For this review, take the finished solid that the model builds, in its own axes (mm). Face numbers are marked on the shaded views. A direction names the side the tool comes from. Coordinates: 2 decimals unless noted, no trailing zeros. Write each loop counter-clockwise with the first axis right and the second up, starting at its lowest first coordinate (ties: lowest second). Pieces come first, ordered by that corner, then holes. Notation, with made-up numbers: M 59,8.25 L 112,8.25 A23 ccw 112,30.25 Z; hole C 69.5,78 d11. An arc over 180 degrees is marked long. One line per question, with ' | ' between items.
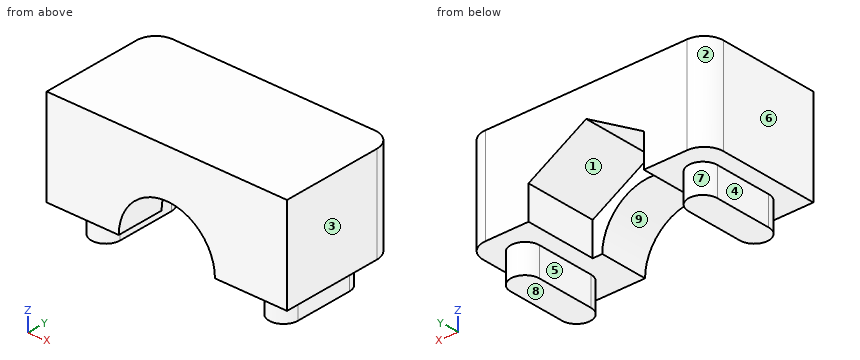
from build123d import *

# Parameters (mm, degrees)
BOSS_EXTRU_1_DEPTH      = 12.5
BOSS_EXTRU_1_DEPTH_BACK = 12.5
ESQUISSE3_W             = 25
ESQUISSE3_H             = 10
BOSS_EXTRU_2_DEPTH      = 12.5
ENL_V_MAT_EXTRU_3_DEPTH = 7.5
ESQUISSE5_R             = 5
ENL_V_MAT_EXTRU_4_DEPTH = 6
ESQUISSE6_W             = 73.841898386
ESQUISSE6_H             = 62.78176119
ENL_V_MAT_EXTRU_5_DEPTH = 26
BOSS_EXTRU_3_DEPTH      = 3
CONG_1_R                = 2


with BuildPart() as part:
    # Esquisse1 → Boss.-Extru.1 (new body, two sides)
    with BuildSketch(Plane(origin=(0, 0, 0), x_dir=(1, 0, 0), z_dir=(0, 1, 0))) as boss_extru_1_sk:
        with BuildLine():
            Line((-3, 21), (-3, -21))
            ThreePointArc((-3, -21), (-4.464466094, -24.535533906), (-8, -26))
            Line((-8, -26), (-63, -26))
            Line((-63, -26), (-63, -29))
            Line((-63, -29), (-3, -29))
            Line((-3, -29), (0, -29))
            Line((0, -29), (0, 29))
            Line((0, 29), (-3, 29))
            Line((-3, 29), (-63, 29))
            Line((-63, 29), (-63, 26))
            Line((-63, 26), (-8, 26))
            ThreePointArc((-8, 26), (-4.464466094, 24.535533906), (-3, 21))
        make_face()
    extrude(amount=BOSS_EXTRU_1_DEPTH)
    extrude(boss_extru_1_sk.sketch, amount=-BOSS_EXTRU_1_DEPTH_BACK)

    # Esquisse3 → Boss.-Extru.2 (add)
    with BuildSketch(Plane(origin=(0, 0, 0), x_dir=(1, 0, 0), z_dir=(0, 1, 0))):
        with Locations((-12.5, 34)):
            Rectangle(ESQUISSE3_W, ESQUISSE3_H)
    extrude(amount=-BOSS_EXTRU_2_DEPTH)

    # Esquisse4 → Enl_v. mat.-Extru.3 (cut)
    with BuildSketch(Plane(origin=(0, 0, 0), x_dir=(1, 0, 0), z_dir=(0, 1, 0))):
        Polygon((-18.5, 39), (-6.5, 44), (-6.5, 35.535898385), (-12.5, 32.07179677), (-18.5, 35.535898385), align=None)
    extrude(amount=-ENL_V_MAT_EXTRU_3_DEPTH, mode=Mode.SUBTRACT)

    # Esquisse5 → Enl_v. mat.-Extru.4 (cut, through all)
    with BuildSketch(Plane(origin=(0, -7.5, 0), x_dir=(1, 0, 0), z_dir=(0, 1, 0))):
        with Locations((-12.5, 39)):
            Circle(ESQUISSE5_R)
    extrude(amount=-ENL_V_MAT_EXTRU_4_DEPTH, mode=Mode.SUBTRACT)

    # Esquisse6 → Enl_v. mat.-Extru.5 (cut, through all)
    with BuildSketch(Plane(origin=(0, 12.5, 0), x_dir=(1, 0, 0), z_dir=(0, 1, 0))):
        with Locations((-26.079050807, -2.390880595)):
            Rectangle(ESQUISSE6_W, ESQUISSE6_H)
    extrude(amount=-ENL_V_MAT_EXTRU_5_DEPTH, mode=Mode.SUBTRACT)

    # Esquisse7 → Boss.-Extru.3 (add)
    with BuildSketch(Plane(origin=(0, 0, -39), x_dir=(-1, 0, 0), z_dir=(0, 0, -1))):
        with BuildLine():
            Line((4.75, -3.25), (4.75, -9.25))
            ThreePointArc((4.75, -9.25), (3.25, -10.75), (1.75, -9.25))
            Line((1.75, -9.25), (1.75, -3.25))
            ThreePointArc((1.75, -3.25), (3.25, -1.75), (4.75, -3.25))
        make_face()
        with BuildLine():
            Line((20.25, -3.25), (20.25, -9.25))
            ThreePointArc((20.25, -9.25), (21.75, -10.75), (23.25, -9.25))
            Line((23.25, -9.25), (23.25, -3.25))
            ThreePointArc((23.25, -3.25), (21.75, -1.75), (20.25, -3.25))
        make_face()
    extrude(amount=BOSS_EXTRU_3_DEPTH)

    # Cong_1
    cong_1_edges = [part.edges().sort_by_distance(p)[0] for p in [
        (-25, 0, -34),
        (0, 0, -34),
    ]]
    fillet(cong_1_edges, radius=CONG_1_R)


solid = part.part
1) Insertion check: pin 1 Ø1.5 at (y, z) = (-6, -41) entering from -X; pin 2 Ø0.9 at (y, z) = (-5, -41) entering from +X; pin 3 Ø4 at (x, z) = (-15, -40.5) entering from +Y. Each pin has a flat end and moves straight along its axis. Give the tip position at first contact, or say it passes through.
Responses:
pin 1: x = -23.25 | pin 2: x = -1.75 | pin 3: through
2) We need section C-C on z = -34.5. State the section outline as (x, y) points, then the cut area to 3 significant figures.
Responses:
outline: M -25,-12.5 L -14.68,-12.5 L -14.68,-7.5 L -16.71,-7.5 L -16.71,0 L -23,0 A2 ccw -25,-2 Z; M -10.32,-12.5 L 0,-12.5 L 0,-2 A2 ccw -2,0 L -8.29,0 L -8.29,-7.5 L -10.32,-7.5 Z | area: 226 mm^2
3) We need section B-B on x = -3.25. State the section outline as (y, z) points.
Responses:
outline: M -12.5,-39 L -10.75,-39 L -10.75,-42 L -1.75,-42 L -1.75,-39 L 0,-39 L 0,-29 L -12.5,-29 Z
4) We need section A-A on y = -7.25. State the section outline as (x, z) points.
Responses:
outline: M -25,-39 L -23.25,-39 L -23.25,-42 L -20.25,-42 L -20.25,-39 L -18.5,-39 L -18.5,-35.54 L -12.5,-32.07 L -6.5,-35.54 L -6.5,-39 L -4.75,-39 L -4.75,-42 L -1.75,-42 L -1.75,-39 L 0,-39 L 0,-29 L -25,-29 Z
5) Machinability: for the marked faces 1, 2, 3, 4 and 5, which of the approach directions +Z, -Z, +X, -X, +Y, -Y give a long, thin tool a straight path to every point of the face, cutting with its end or side? Answer none if there is none.
Responses:
face 1: -Z, +Y | face 2: +Z, -Z, -X, +Y | face 3: +Z, -Z, +X, +Y, -Y | face 4: -Z, -X, +Y, -Y | face 5: -Z, +Y, -Y
6) To check wall thickness, follow line 1 along X through (y, z) = (-8, -40); line 2 along X through (y, z) = (-3.25, -38.5); line 3 along Z through (x, y) = (-21.75, -0.5). State the ranges of each line that lie inside material, in increasing order. Write a range as [from, to].
Responses:
line 1: [-23.25, -20.25], [-4.75, -1.75] | line 2: [-25, -18.5], [-6.5, 0] | line 3: [-39, -29]
7) We need section D-D on y = -8.75. State the section outline as (x, z) points, then the cut area to 3 significant figures.
Responses:
outline: M -25,-39 L -23.25,-39 L -23.25,-42 L -20.25,-42 L -20.25,-39 L -17.5,-39 A5 cw -7.5,-39 L -4.75,-39 L -4.75,-42 L -1.75,-42 L -1.75,-39 L 0,-39 L 0,-29 L -25,-29 Z | area: 229 mm^2
8) The part is to be moulded in two halves that separate along X. For the marked faces 6, 7, 8 and 9, say which applies: +X half, -X half, draft (parallel to the pull), parting line (faces both ways), or undercut.
Responses:
face 6: -X half | face 7: undercut | face 8: draft | face 9: undercut
